Autodesk Inventor part; units mm, degrees
ref_plane "YZ Plane" through (0, 0, 0) normal (1, 0, 0) x (0, 1, 0)
ref_plane "XZ Plane" through (0, 0, 0) normal (0, 1, 0) x (-1, 0, 0)
ref_plane "XY Plane" through (0, 0, 0) normal (0, 0, 1) x (1, 0, 0)
sketch "Sketch1" plane through (0, 0, 0) normal (0, 1, 0) x (-1, 0, 0)
  circle A0 centre (0, -5.8) radius 1.45
  circle A1 centre (0, 0) radius 1.45
  line L0 (-1.45, -5.923) -> (-1.45, 0.123)
  line L1 (1.45, 0.123) -> (1.45, -5.923)
  circle A2 centre (0, -5.8) radius 1.45
  circle A3 centre (0, 0) radius 1.45
  line L2 (-1.45, -5.923) -> (-1.45, 0.123)
  line L3 (1.45, -5.923) -> (1.45, 0.123)
  line L4 (-1.45, -5.923) -> (1.45, -0.0104)
  line L5 (1.45, -5.923) -> (-1.45, -0.0056)
  line L6 (5.87, 3.81) -> (-3.02, 3.81)
  line L7 (-3.02, 3.81) -> (-3.02, -9.3582)
  line L8 (5.87, -9.3582) -> (5.87, 3.81)
  line L9 (0, -5.8) -> (0, -9.61)
  line L10 (5.87, -9.3582) -> (5.87, -9.61)
  line L11 (5.87, -9.61) -> (0, -9.61)
  line L12 (-3.02, -9.61) -> (-3.02, -9.3582)
  line L13 (0, -9.61) -> (-3.02, -9.61)
  point P0 (3.8566, 2.9938)
  point P1 (-1.4456, -5.9139)
  point P2 (-1.45, -5.8099)
  point P3 (-1.45, -5.7901)
  point P4 (-1.45, -0.0056)
  point P5 (1.45, -0.0104)
  point P6 (1.45, -5.7873)
  point P7 (1.45, -5.8126)
  point P8 (1.4456, -5.9139)
  dimension "d4" = 0
  dimension "d5" = 2.9
  dimension "d6" = 2.9001
  dimension "d8" = 1.57
  dimension "d9" = 8.89
  dimension "d11" = 3.81
  dimension "d13" = 3.81
extrude "Extrusion1" add sketch "Sketch1" along normal blind 1.27
sketch "Sketch2" plane through (3.02, 0, 3.81) normal (1, 0, 0) x (0, 0, -1)
  line L0 (9.6001, 1.27) -> (3.8156, 1.27)
  line L1 (3.8204, 1.27) -> (9.5973, 1.27)
  line L2 (2.36, 1.27) -> (3.8204, 1.27)
  line L3 (9.7239, 1.27) -> (11.06, 1.27)
  line L4 (6.71, 0) -> (6.71, 13.97)
  line L5 (6.71, 13.97) -> (21.95, 13.97)
  line L6 (21.95, 13.97) -> (21.95, 0)
  line L7 (21.95, 0) -> (6.71, 0)
  line L8 (6.71, 0) -> (6.71, 13.97)
  line L9 (6.71, 13.97) -> (-8.53, 13.97)
  line L10 (-8.53, 13.97) -> (-8.53, 0)
  line L11 (-8.53, 0) -> (6.71, 0)
  line L12 (6.71, 0) -> (6.71, 13.97)
  line L13 (0, 0) -> (13.42, 0)
  line L14 (13.42, 0) -> (13.42, 1.27)
  line L15 (0, 1.27) -> (13.42, 1.27)
  line L16 (0, 0) -> (0, 1.27)
  circle A0 centre (14.33, 2.5137) radius 1.5
  circle A1 centre (-0.91, 2.5137) radius 1.5
  point P0 (3.81, 0)
  point P1 (9.7239, 1.27)
  dimension "d19" = 15.24
  dimension "d20" = 15.24
  dimension "d21" = 7.62
  dimension "d22" = 7.62
  dimension "d23" = 3
  dimension "d24" = 3
extrude "Extrusion2" add sketch "Sketch2" along normal blind 2.54
properties part number "USB_MOUNT"
Source: CAD feature listing. Evaluate the final solid. Frame: model axes, mm. A direction names the side the tool comes from. Round coordinates to 2 decimals unless told otherwise and drop trailing zeros. Loops run counter-clockwise (first coordinate to the right, second up) from the corner with the lowest first, then second, coordinate; pieces in that order, holes last.
(1) Access query for faces 1 (the flat face through (-1, 1, 3.81)), 2 (the flat face through (-1, 1, -9.61)), 3 (the flat face through (-2, 1.27, -3)), 4 (the flat face through (1.45, 1, -3)). Directions: +Z, -Z, +X, -X, +Y, -Y. A direction counts if a zero-diameter tool reaches every point of the face in a straight line with its end or side. Return the directions, or none.
From the geometry:
face 1: +Z, -X, +Y, -Y
face 2: -Z, -X, +Y, -Y
face 3: +Z, -Z, -X, +Y
face 4: +Y, -Y
(2) Pull-direction query (X, two-part tool) for faces 5 (the flat face through (4, 7, -18.14)), 6 (the cylindrical face through (-0.03, 0.63, -7.25)), 7 (the flat face through (5.56, 7, -3)); classes: +X half, -X half, draft (parallel to the pull), parting line (faces both ways), or undercut.
From the geometry:
face 5: draft
face 6: undercut
face 7: +X half
(3) Contact query for flat-ended pins moving along their axis: pin 1 Ø3 at (x, y) = (0.5, 5.5) entering from -Z; pin 2 Ø0.6 at (x, y) = (-2, 0.5) entering from +Z; pin 3 Ø2 at (y, z) = (1.5, -14) entering from -X; pin 4 Ø1 at (x, y) = (0.5, 0.5) entering from -Z. Output: stop coordinate, or through.
From the geometry:
pin 1: passes through
pin 2: stops at z = 3.81
pin 3: stops at x = 3.02
pin 4: stops at z = -9.61
(4) Section query B-B (x = 1). Output: boundary loops of the cut face in (y, z).
From the geometry:
outline: (0, -9.61) - (1.27, -9.61) - (1.27, -6.85) - (0, -6.85) - close; (0, 1.05) - (1.27, 1.05) - (1.27, 3.81) - (0, 3.81) - close
(5) Material intervals for probe 1 along Y at (x, z) = (4.2, -10.52); probe 2 along Y at (x, z) = (-2.75, -8.5); probe 3 along Z at (x, y) = (4.5, 3), sorted ascending.
From the geometry:
probe 1: y = 0 to 1.01, 4.01 to 13.97
probe 2: y = 0 to 1.27
probe 3: z = -18.14 to -11.94, -9.1 to 3.3, 6.14 to 12.34
(6) Section query C-C (z = -10.52). Output: boundary loops of the cut face in (x, y), and give its area (3 significant figures).
From the geometry:
outline: (3.02, 0) - (5.56, 0) - (5.56, 1.01) - (3.02, 1.01) - close; (3.02, 4.01) - (5.56, 4.01) - (5.56, 13.97) - (3.02, 13.97) - close
area: 27.9 mm2
(7) Section query A-A (z = 1). Output: boundary loops of the cut face in (x, y), and give its area (3 significant figures).
From the geometry:
outline: (-5.87, 0) - (-1.05, 0) - (-1.05, 1.27) - (-5.87, 1.27) - close; (1.05, 0) - (5.56, 0) - (5.56, 13.97) - (3.02, 13.97) - (3.02, 1.27) - (1.05, 1.27) - close
area: 44.1 mm2
(8) Section query D-D (y = 10.25). Output: boundary loops of the cut face in (x, z).
From the geometry:
outline: (3.02, -18.14) - (5.56, -18.14) - (5.56, 12.34) - (3.02, 12.34) - close
